Geometry check sheet. Reference: the model listing, model coordinates, mm. Face numbers are marked on the shaded views. A direction names the side the tool comes from. Round coordinates to 2 decimals unless told otherwise and drop trailing zeros. Loops run counter-clockwise (first coordinate to the right, second up) from the corner with the lowest first, then second, coordinate; pieces in that order, holes last. Notation, with made-up numbers: M 65,19 L 79,19 A18 cw 79,37 Z; hole C 52.5,58.5 d5. An arc over 180 degrees is marked long. Answer in a Markdown table with one row per item. Add a question column.
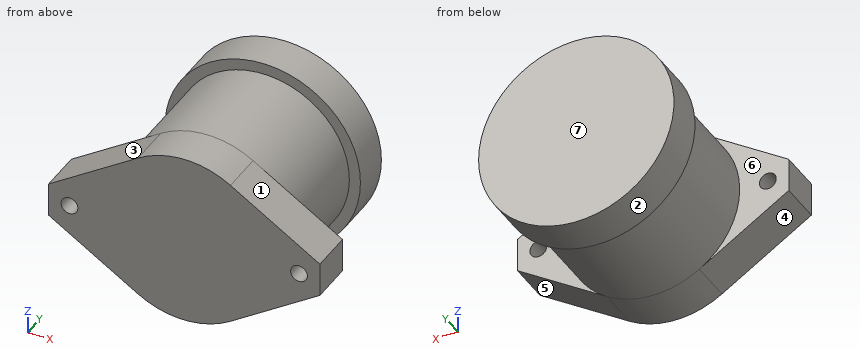
```python
from build123d import *

# Parameters (mm, degrees)
SKETCH1_R           = 2.5
BOSS_EXTRUDE1_DEPTH = 12.954
SKETCH2_R           = 25.781
BOSS_EXTRUDE2_DEPTH = 43.942
SKETCH3_R           = 29.083
BOSS_EXTRUDE3_DEPTH = 12


with BuildPart() as part:
    # Sketch1 → Boss-Extrude1 (new body)
    with BuildSketch(Plane(origin=(0, 0, 0), x_dir=(1, 0, 0), z_dir=(0, 1, 0))):
        with BuildLine():
            Line((-40.386, -5), (-40.386, 5))
            Line((-40.386, 5), (-13.758365761, 21.802920277))
            ThreePointArc((-13.758365761, 21.802920277), (0, 25.781), (13.758365761, 21.802920277))
            Line((13.758365761, 21.802920277), (40.386, 5))
            Line((40.386, 5), (40.386, -5))
            Line((40.386, -5), (13.758365761, -21.802920277))
            ThreePointArc((13.758365761, -21.802920277), (0, -25.781), (-13.758365761, -21.802920277))
            Line((-13.758365761, -21.802920277), (-40.386, -5))
        make_face()
        with Locations((-34.163, 0)):
            Circle(SKETCH1_R, mode=Mode.SUBTRACT)
        with Locations((34.163, 0)):
            Circle(SKETCH1_R, mode=Mode.SUBTRACT)
    extrude(amount=BOSS_EXTRUDE1_DEPTH)

    # Sketch2 → Boss-Extrude2 (add)
    with BuildSketch(Plane(origin=(0, 12.954, 0), x_dir=(1, 0, 0), z_dir=(0, 1, 0))):
        Circle(SKETCH2_R)
    extrude(amount=BOSS_EXTRUDE2_DEPTH)

    # Sketch3 → Boss-Extrude3 (add)
    with BuildSketch(Plane(origin=(0, 56.896, 0), x_dir=(1, 0, 0), z_dir=(0, 1, 0))):
        Circle(SKETCH3_R)
    extrude(amount=-BOSS_EXTRUDE3_DEPTH)


solid = part.part
```
1) Draft check along Y on the marked faces 5, 6 and 7. Enter one of: +Y half, -Y half, draft (parallel to the pull), parting line (faces both ways), or undercut.
2) Cross-section at C-C, the plane x = 0.5. Record the boundary of the cut face in (y, z), plus the area to 3 significant figures.
3) Thickness scan on L1, parallel to X at y = 5, z = 0; L2, parallel to X at y = 46.5, z = 11; L3, parallel to X at y = 41.5, z = 16.5. Record the ranges inside material, lowest first. Write a range as [from, to].
4) Set-up check for the marked faces 1, 2, 3 and 4: record each of +Z, -Z, +X, -X, +Y, -Y from which the full face is reachable in a straight line by a thin tool's end or side.
5) Go/stop test with flat-tipped pins: pin 1 (8 mm diameter, centred on x = 11.5, y = 38, fed in from +Z); pin 2 (2 mm diameter, centred on x = 7, y = 26.5, fed in from -Z); pin 3 (1.5 mm diameter, centred on x = 4, y = 36, fed in from +Z). Record where each tip stops, or that it passes through.
6) Cross-section at B-B, the plane z = 0. Record the boundary of the cut face in (x, y).
7) Cross-section at D-D, the plane z = 16. Record the boundary of the cut face in (x, y).
8) Cross-section at A-A, the plane y = 6. Record the boundary of the cut face in (x, z).
Worked answers:
| question | item | result |
|---|---|---|
| 1 | face 5 | draft |
| 1 | face 6 | undercut |
| 1 | face 7 | +Y half |
| 2 | outline | M 0,-25.78 L 44.9,-25.78 L 44.9,-29.08 L 56.9,-29.08 L 56.9,29.08 L 44.9,29.08 L 44.9,25.78 L 0,25.78 Z |
| 2 | area | 3,010 mm2 |
| 3 | L1 | x = [-40.39, -36.66], [-31.66, 31.66], [36.66, 40.39] |
| 3 | L2 | x = [-26.92, 26.92] |
| 3 | L3 | x = [-19.81, 19.81] |
| 4 | face 1 | +Z, +X, -Y |
| 4 | face 2 | +Y |
| 4 | face 3 | +Z, -X, -Y |
| 4 | face 4 | -Z, -X, -Y |
| 5 | pin 1 | stops at z = 24.67 |
| 5 | pin 2 | stops at z = -25.07 |
| 5 | pin 3 | stops at z = 25.58 |
| 6 | outline | M -40.39,0 L -36.66,0 L -36.66,12.95 L -40.39,12.95 Z; M -31.66,0 L 31.66,0 L 31.66,12.95 L 25.78,12.95 L 25.78,44.9 L 29.08,44.9 L 29.08,56.9 L -29.08,56.9 L -29.08,44.9 L -25.78,44.9 L -25.78,12.95 L -31.66,12.95 Z; M 36.66,0 L 40.39,0 L 40.39,12.95 L 36.66,12.95 Z |
| 7 | outline | M -24.29,44.9 L -20.22,44.9 L -20.22,12.95 L -22.95,12.95 L -22.95,0 L 22.95,0 L 22.95,12.95 L 20.22,12.95 L 20.22,44.9 L 24.29,44.9 L 24.29,56.9 L -24.29,56.9 Z |
| 8 | outline | M -40.39,-5 L -13.76,-21.8 A25.78 ccw 13.76,-21.8 L 40.39,-5 L 40.39,5 L 13.76,21.8 A25.78 ccw -13.76,21.8 L -40.39,5 Z; hole C -34.16,0 d5; hole C 34.16,0 d5 |
